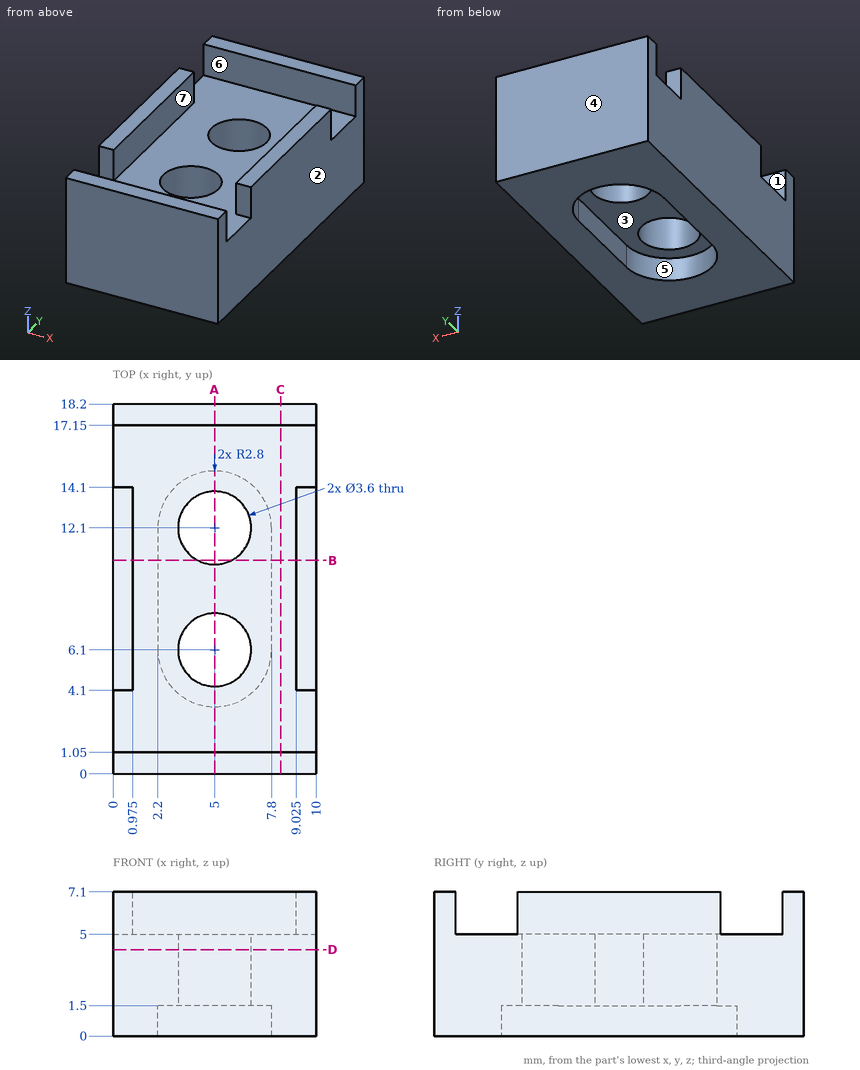
Print and shaded views of the part. All mm, measured from the part's lowest x, y and z. A direction names the side the tool comes from. Give positions to 0.01 mm unless a question says otherwise; leave off trailing zeros. Loops run counter-clockwise (first coordinate to the right, second up) from the corner with the lowest first, then second, coordinate; pieces in that order, holes last.
1) Saw through at D-D (z = 4.25). Write the cut outline in (x, y), plus the area to 3 significant figures.
2) Saw through at A-A (x = 5). Write the cut outline in (y, z), plus the area to 3 significant figures.
3) Tool access for the marked faces 4, 5, 6 and 7: list every direction of +Z, -Z, +X, -X, +Y, -Y with a clear straight run to the whole face (end or side of a thin tool).
4) Saw through at C-C (x = 8.25). Write the cut outline in (y, z), plus the area to 3 significant figures.
5) Pull direction X, two halves, no side cores. Call the marked faces 1, 2 and 3: +X half, -X half, draft (parallel to the pull), parting line (faces both ways), or undercut.
6) Wall check: line 1 (Y direction, x = 5, z = 3.6); line 2 (Y direction, x = 1.25, z = 5.25); line 3 (Y direction, x = 6.5, z = 3.25). Give the ranges that are in metal, low to high.
7) Saw through at B-B (y = 10.5). Write the cut outline in (x, z) (3 decimals), plus the area to 3 significant figures.
8) Flat gauge pins, fed straight in: pin 1 Ø1 at (x, y) = (3.5, 5.5) entering from +Z; pin 2 Ø1.7 at (x, y) = (4, 10) entering from -Z; pin 3 Ø3 at (x, y) = (5, 6.1) entering from +Z. Where does each tip first touch, or does it go through?
Answer block:
1. outline: (0, 0) - (10, 0) - (10, 18.2) - (0, 18.2) - close; hole circle Ø3.6 at (5, 6.1); hole circle Ø3.6 at (5, 12.1)
1. area: 162 mm2
2. outline: (0, 0) - (3.3, 0) - (3.3, 1.5) - (4.3, 1.5) - (4.3, 5) - (1.05, 5) - (1.05, 7.1) - (0, 7.1) - close; (7.9, 1.5) - (10.3, 1.5) - (10.3, 5) - (7.9, 5) - close; (13.9, 1.5) - (14.9, 1.5) - (14.9, 0) - (18.2, 0) - (18.2, 7.1) - (17.15, 7.1) - (17.15, 5) - (13.9, 5) - close
2. area: 52.8 mm2
3. face 4: +Z, -Z, +X, -X, +Y
3. face 5: -Z
3. face 6: +Z, +X, -X
3. face 7: +Z
4. outline: (0, 0) - (18.2, 0) - (18.2, 7.1) - (17.15, 7.1) - (17.15, 5) - (1.05, 5) - (1.05, 7.1) - (0, 7.1) - close
4. area: 95.4 mm2
5. face 1: draft
5. face 2: +X half
5. face 3: undercut
6. line 1: y = 0 to 4.3, 7.9 to 10.3, 13.9 to 18.2
6. line 2: y = 0 to 1.05, 17.15 to 18.2
6. line 3: y = 0 to 5.11, 7.09 to 11.11, 13.09 to 18.2
7. outline: (0, 0) - (2.2, 0) - (2.2, 1.5) - (4.175, 1.5) - (4.175, 5) - (0.975, 5) - (0.975, 7.1) - (0, 7.1) - close; (5.825, 1.5) - (7.8, 1.5) - (7.8, 0) - (10, 0) - (10, 7.1) - (9.025, 7.1) - (9.025, 5) - (5.825, 5) - close
7. area: 39.9 mm2
8. pin 1: stops at z = 5
8. pin 2: stops at z = 1.5
8. pin 3: passes through
